Read the model definition and answer for the solid it produces. Units are mm, in the model's axes. A direction names the side the tool comes from. Coordinates: 2 decimals unless noted, no trailing zeros. Write each loop counter-clockwise with the first axis right and the second up, starting at its lowest first coordinate (ties: lowest second). Pieces come first, ordered by that corner, then holes.
Item 1: A tool of negligible diameter and unlimited length cuts with its end or side. For faces 4 (the face through (61, 2, -7)), 5 (the face through (71, 0, -7)), from which of +Z, -Z, +X, -X, +Y, -Y can it reach the whole face along a straight path? Write none if from no direction.
Item 2: Section D-D (x = 46) is taken. Give the vertices of the cut face in (y, z).
Item 3: Section B-B (z = -13.5) is taken. Give the vertices of the cut face in (x, y).
Item 4: Each of these flat-tipped pins is pushed along its axis until it touches: P1, Ø6, axis at y = 17, z = -11.5, coming from the -X side; P2, Ø5, axis at x = 6, y = 5, coming from the -Z side; P3, Ø1.5, axis at x = 42, z = -3.5, coming from the +Y side; P4, Ø1.5, axis at y = 4.5, z = -5, coming from the +X side. Where does it stop, or does it pass through?
Item 5: Section C-C (y = 3.25) is taken. Give the vertices of the cut face in (x, z).
Item 6: Determine the mould class of faces 1 (the face through (31.36, 29.69, -7.4)), 2 (the face through (30, 18, -15)), 3 (the face through (0, 2, -7)) for opening direction X: released by +X, released by -X, zero draft, split by the parting line, or undercut.
Item 7: Straight lines are drawn through the part: probe 1 along X at (y, z) = (6.75, -3.5); probe 2 along X at (y, z) = (4.5, -4.25); probe 3 along X at (y, z) = (21, -7.25). For each, find the intervals that lie inside material, in ascending order.
Item 8: Section A-A (y = 11.25) is taken. Give the vertices of the cut face in (x, z).
Solid Edge part; units mm, degrees
sketch "Sketch1" plane through (0, 0, 0) normal (0, 0, 1) x (1, 0, 0)
  line L0 (0, 0) -> (0, 5)
  arc A0 (61, 5) -> (0, 5) centre (30.5, -28.087) ccw
  line L1 (61, 0) -> (61, 5)
  line L2 (61, 0) -> (81, 0)
  arc A1 (81, 0) -> (-20, 0) centre (30.5, -28.087) ccw
  line L3 (0, 0) -> (-20, 0)
  dimension "D1" = 61
  dimension "D2" = 61
extrude "Protrusion1" add sketch "Sketch1" against normal blind 15
properties material "Aluminum, 6061-T6"
Established:
1. face 4: +Z, -Z, -Y
1. face 5: +Z, -Z, +X, -X, -Y
2. outline: (14.16, -15) - (27.58, -15) - (27.58, 0) - (14.16, 0) - close
3. outline: (-20, 0) - (0, 0) - (0, 5) arc R45 cw to (61, 5) - (61, 0) - (81, 0) arc R57.79 ccw to start
4. P1: stops at x = -9.1
4. P2: passes through
4. P3: stops at y = 28.69
4. P4: stops at x = 78.72
5. outline: (-18.05, -15) - (0, -15) - (0, 0) - (-18.05, 0) - close; (61, -15) - (79.05, -15) - (79.05, 0) - (61, 0) - close
6. face 1: split by the parting line
6. face 2: zero draft
6. face 3: undercut
7. probe 1: x = -15.6 to 2.02, 58.98 to 76.6
7. probe 2: x = -17.22 to 0, 61 to 78.22
7. probe 3: x = 0.01 to 60.99
8. outline: (-11.83, -15) - (8.65, -15) - (8.65, 0) - (-11.83, 0) - close; (52.35, -15) - (72.83, -15) - (72.83, 0) - (52.35, 0) - close
